```python
from build123d import *

# Parameters (mm, degrees)
F0_W     = 18
F0_H     = 15
F1_DEPTH = 15
F3_DEPTH = 25
F4_W     = 10
F4_H     = 15
F5_DEPTH = 10
F7_DEPTH = 25
F9_DEPTH = 2
F10_R    = 1


with BuildPart() as f1:
    # F0 (on Top) → F1 (new body)
    with BuildSketch(Plane.XY):
        with Locations((9, 7.5)):
            Rectangle(F0_W, F0_H)
    extrude(amount=F1_DEPTH)

    # F2 (on face) → F3 (cut)
    with BuildSketch(Plane(origin=(0, 0, 0), x_dir=(0, -1, 0), z_dir=(-1, 0, 0))):
        with BuildLine():
            Line((-11, 7.95), (-4, 7.95))
            ThreePointArc((-4, 7.95), (-1.95, 10), (-4, 12.05))
            Line((-4, 12.05), (-11, 12.05))
            ThreePointArc((-11, 12.05), (-13.05, 10), (-11, 7.95))
        make_face()
    extrude(amount=-F3_DEPTH, mode=Mode.SUBTRACT)

    # F4 (on face) → F5 (cut)
    with BuildSketch(Plane.XY.offset(15)):
        with Locations((13, 7.5)):
            Rectangle(F4_W, F4_H)
    extrude(amount=-F5_DEPTH, mode=Mode.SUBTRACT)

    # F6 (on face) → F7 (cut)
    with BuildSketch(Plane.XY.offset(5)):
        with BuildLine():
            Line((15.05, 4), (15.05, 11))
            ThreePointArc((15.05, 11), (13, 13.05), (10.95, 11))
            Line((10.95, 11), (10.95, 4))
            ThreePointArc((10.95, 4), (13, 1.95), (15.05, 4))
        make_face()
    extrude(amount=-F7_DEPTH, mode=Mode.SUBTRACT)

    # F8 (on face) → F9 (cut)
    with BuildSketch(Plane.XY.offset(5)):
        with BuildLine():
            Line((16, 4), (16, 11))
            ThreePointArc((16, 11), (13, 14), (10, 11))
            Line((10, 11), (10, 4))
            ThreePointArc((10, 4), (13, 1), (16, 4))
        make_face()
    extrude(amount=-F9_DEPTH, mode=Mode.SUBTRACT)

    # F10
    f10_edges = [f1.edges().sort_by_distance(p)[0] for p in [
        (8, 7.5, 5),
    ]]
    fillet(f10_edges, radius=F10_R)


solid = f1.part
```
Design review of the part built by this model. Coordinates are the model's own, in mm. A direction names the side the tool comes from. Round coordinates to 2 decimals unless told otherwise and drop trailing zeros. Order: outer loops, then holes, each group sorted by start corner. A loop starts at its lowest first (then second) coordinate and runs counter-clockwise, first axis right, second up. Notation, with made-up numbers: (1.25, 77) - (42.25, 77) arc R17 ccw to (42.25, 84) - close; hole circle Ø3 at (44.25, 17). An arc over 180 degrees is marked (long way). Return JSON: item names as keys, results as strings.
Q1. For pin 1 Ø5 at (x, y) = (14.5, 8) entering from +Z; pin 2 Ø5 at (y, z) = (5.5, 11.5) entering from +X, all flat-tipped, find the tip position at first contact; note any pin that passes through.
Computed values:
{"pin 1": "stops at z = 5", "pin 2": "stops at x = 8"}
Q2. Wall thickness on L1, parallel to X at y = 10.25, z = 2.5; L2, parallel to Z at x = 3.75, y = 5.5; L3, parallel to Y at x = 13, z = 4: over which ranges is each line inside the solid? List them lowest first. Write a range as [from, to].
Computed values:
{"L1": "x = [0, 10.95], [15.05, 18]", "L2": "z = [0, 7.95], [12.05, 15]", "L3": "y = [0, 1], [14, 15]"}
Q3. Consider section D-D on x = 6. Write out the cut boundary in (y, z), plus the area to 3 significant figures.
Computed values:
{"outline": "(0, 0) - (15, 0) - (15, 15) - (0, 15) - close; hole (4, 7.95) - (11, 7.95) arc R2.05 ccw to (11, 12.05) - (4, 12.05) arc R2.05 ccw to start", "area": "183 mm2"}
Q4. Consider section A-A on y = 9.5. Write out the cut boundary in (x, z), plus the area to 3 significant figures.
Computed values:
{"outline": "(0, 0) - (10.95, 0) - (10.95, 3) - (10, 3) - (10, 5) - (9, 5) arc R1 cw to (8, 6) - (8, 7.95) - (0, 7.95) - close; (0, 12.05) - (8, 12.05) - (8, 15) - (0, 15) - close; (15.05, 0) - (18, 0) - (18, 5) - (16, 5) - (16, 3) - (15.05, 3) - close", "area": "113 mm2"}
Q5. Consider section B-B on x = 13. Write out the cut boundary in (y, z), plus the area to 3 significant figures.
Computed values:
{"outline": "(0, 0) - (1.95, 0) - (1.95, 3) - (1, 3) - (1, 5) - (0, 5) - close; (13.05, 0) - (15, 0) - (15, 5) - (14, 5) - (14, 3) - (13.05, 3) - close", "area": "15.7 mm2"}
Q6. Machinability: for faces 4 (the flat face through (8, 7, 13)), 5 (the flat face through (4, 8, 7.95)), 6 (the flat face through (10.3, 7.6, 3)), which of the approach directions +Z, -Z, +X, -X, +Y, -Y give a long, thin tool a straight path to every point of the face, cutting with its end or side? Answer none if there is none.
Computed values:
{"face 4": "+Z, +X, +Y, -Y", "face 5": "+X, -X", "face 6": "+Z"}
Q7. The part is to be moulded in two halves that separate along X. For faces 1 (the flat face through (18, 7, 2)), 2 (the flat face through (4, 7, 12.05)), 3 (the flat face through (15.05, 7, 2)), say which applies: pulls with the +X half, pulls with the -X half, needs draft (parallel to the pull), parting line crosses it, or undercut.
Computed values:
{"face 1": "pulls with the +X half", "face 2": "needs draft", "face 3": "undercut"}
Q8. Consider section C-C on z = 10. Write out the cut boundary in (x, y).
Computed values:
{"outline": "(0, 0) - (8, 0) - (8, 1.95) - (0, 1.95) - close; (0, 13.05) - (8, 13.05) - (8, 15) - (0, 15) - close"}
